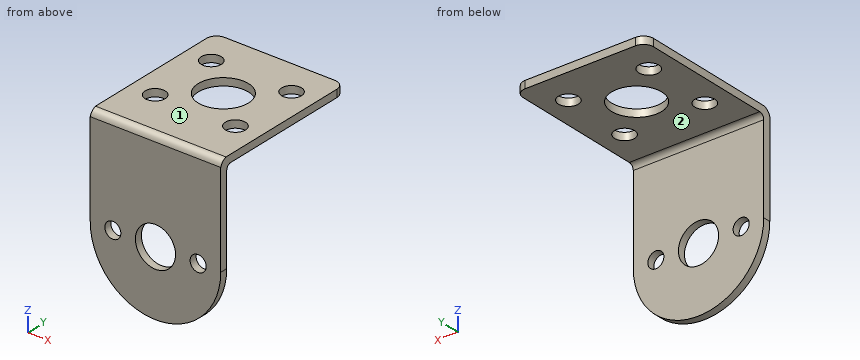
```python
from build123d import *

# Parameters (mm, degrees)
SKETCH1_R           = 40
SKETCH1_R_2         = 16
BOSS_EXTRUDE1_DEPTH = 15
SKETCH2_R           = 50
SKETCH2_R_2         = 20
BOSS_EXTRUDE2_DEPTH = 15
CUT_EXTRUDE2_START  = -260
CUT_EXTRUDE2_DEPTH  = 260
FILLET1_R           = 10
SCALE2_SCALE        = 0.1


# Read off the part's stored shape, not the designer's step: Cut-Extrude2
with BuildPart() as part:
    # Sketch1 → Boss-Extrude1 (new body)
    with BuildSketch(Plane(origin=(0, 0, 0), x_dir=(1, 0, 0), z_dir=(0, 1, 0))):
        with BuildLine():
            Line((-130, -200), (-130, 0))
            ThreePointArc((-130, 0), (0, 130), (130, 0))
            Line((130, 0), (130, -200))
            Line((130, -200), (-130, -200))
        make_face()
        with Locations(Location((0, 0, 0), (0, 0, 270))):
            Circle(SKETCH1_R, mode=Mode.SUBTRACT)
        with Locations(Location((-85, 0, 0), (0, 0, 270))):
            Circle(SKETCH1_R_2, mode=Mode.SUBTRACT)
        with Locations(Location((85, 0, 0), (0, 0, 270))):
            Circle(SKETCH1_R_2, mode=Mode.SUBTRACT)
    extrude(amount=BOSS_EXTRUDE1_DEPTH)

    # Sketch2 → Boss-Extrude2 (add)
    with BuildSketch(Plane.XY.offset(200)):
        with BuildLine():
            Line((-130, 0), (-130, 290))
            ThreePointArc((-130, 290), (-124.142135624, 304.142135624), (-110, 310))
            Line((-110, 310), (110, 310))
            ThreePointArc((110, 310), (124.142135624, 304.142135624), (130, 290))
            Line((130, 290), (130, 0))
            Line((130, 0), (-130, 0))
        make_face()
        with Locations((0, 169.361818375)):
            Circle(SKETCH2_R, mode=Mode.SUBTRACT)
        with Locations((80, 239.361818375)):
            Circle(SKETCH2_R_2, mode=Mode.SUBTRACT)
        with Locations((-80, 239.361818375)):
            Circle(SKETCH2_R_2, mode=Mode.SUBTRACT)
        with Locations((-80, 99.361818375)):
            Circle(SKETCH2_R_2, mode=Mode.SUBTRACT)
        with Locations((80, 99.361818375)):
            Circle(SKETCH2_R_2, mode=Mode.SUBTRACT)
    extrude(amount=-BOSS_EXTRUDE2_DEPTH)

    # Cut-Extrude2 outline → Cut-Extrude2 (cut)
    with BuildSketch(Plane.ZY.offset(130).offset(CUT_EXTRUDE2_START)):
        with BuildLine():
            ThreePointArc((200, 13.029030935), (195.075286181, 4.924713819), (186.970969065, 0))
            Line((186.970969065, 0), (200, 0))
            Line((200, 0), (200, 13.029030935))
        make_face()
    extrude(amount=CUT_EXTRUDE2_DEPTH, mode=Mode.SUBTRACT)

    # Fillet1
    fillet1_edges = [part.edges().sort_by_distance(p)[0] for p in [
        (0, 15, 185),
    ]]
    fillet(fillet1_edges, radius=FILLET1_R)


with BuildPart() as part_1:
    # Scale2: scaled about (0, 79.825718393, 117.542480981)
    add(part.part.scale(SCALE2_SCALE).moved(Location((0, 71.843146554, 105.788232883))))


solid = part_1.part
```
Here's how the part is built. I have some questions about the finished solid (model axes, mm). Face numbers are marked on the shaded views. A direction names the side the tool comes from. Coordinates: 2 decimals unless noted, no trailing zeros. Write each loop counter-clockwise with the first axis right and the second up, starting at its lowest first coordinate (ties: lowest second). Pieces come first, ordered by that corner, then holes. Notation, with made-up numbers: (-0.75, 58.25) -> (15.25, 58.25) arc R16 ccw to (15.25, 64.25) -> close; hole circle Ø10 at (55, 77). An arc over 180 degrees is marked (long way). Use a Markdown table: item, result. Add a question column.
(1) If we section it at C-C, the plane z = 106.5: Write out the boundary of the cut face in (x, y), and give its area (3 significant figures).
(2) If we section it at A-A, the plane x = 0: Write out the boundary of the cut face in (y, z), and give its area (3 significant figures).
(3) For the marked faces 1 and 2, which set-ups out of +Z, -Z, +X, -X, +Y, -Y let a thin tool reach every point of the face, with its end or its side?
(4) If we section it at B-B, the plane z = 102.5: Write out the boundary of the cut face in (x, y), and give its area (3 significant figures).
(5) I'm going to push flat-ended pins straight in: P1, Ø5, axis at x = 8, y = 95.78, coming from the -Z side; P2, Ø1, axis at x = 7, z = 119, coming from the +Y side. Where does each tip first touch, or does it pass through?
(6) If we section it at D-D, the plane y = 83: Write out the boundary of the cut face in (x, z).
(7) Please list where these lines run through material, in increasing order: line 1 (Y direction, x = -8, z = 125.35); line 2 (Y direction, x = -8, z = 124.7); line 3 (Z direction, x = 7, y = 98.5).
Outcome:
| question | item | result |
|---|---|---|
| 1 | outline | (-13, 71.84) -> (-9.93, 71.84) -> (-9.93, 73.34) -> (-13, 73.34) -> close; (-7.07, 71.84) -> (-3.94, 71.84) -> (-3.94, 73.34) -> (-7.07, 73.34) -> close; (3.94, 71.84) -> (7.07, 71.84) -> (7.07, 73.34) -> (3.94, 73.34) -> close; (9.93, 71.84) -> (13, 71.84) -> (13, 73.34) -> (9.93, 73.34) -> close |
| 1 | area | 18.6 mm^2 |
| 2 | outline | (71.84, 92.79) -> (73.34, 92.79) -> (73.34, 101.79) -> (71.84, 101.79) -> close; (71.84, 109.79) -> (73.34, 109.79) -> (73.34, 123.29) arc R1 cw to (74.34, 124.29) -> (83.78, 124.29) -> (83.78, 125.79) -> (73.15, 125.79) arc R2 ccw to (71.84, 124.49) -> close; (93.78, 124.29) -> (102.84, 124.29) -> (102.84, 125.79) -> (93.78, 125.79) -> close |
| 2 | area | 66.4 mm^2 |
| 3 | face 1 | +Z, +X, -X, +Y, -Y |
| 3 | face 2 | -Z, +X, -X, +Y |
| 4 | outline | (-12.58, 71.84) -> (-2.28, 71.84) -> (-2.28, 73.34) -> (-12.58, 73.34) -> close; (2.28, 71.84) -> (12.58, 71.84) -> (12.58, 73.34) -> (2.28, 73.34) -> close |
| 4 | area | 30.9 mm^2 |
| 5 | P1 | stops at z = 124.29 |
| 5 | P2 | stops at y = 73.34 |
| 6 | outline | (-13, 124.29) -> (-9.58, 124.29) -> (-9.58, 125.79) -> (-13, 125.79) -> close; (-6.42, 124.29) -> (6.42, 124.29) -> (6.42, 125.79) -> (-6.42, 125.79) -> close; (9.58, 124.29) -> (13, 124.29) -> (13, 125.79) -> (9.58, 125.79) -> close |
| 7 | line 1 | y = 72.39 to 79.78, 83.78 to 93.78, 97.78 to 102.84 |
| 7 | line 2 | y = 71.92 to 79.78, 83.78 to 93.78, 97.78 to 102.84 |
| 7 | line 3 | z = 124.29 to 125.79 |
